Work out the finished part from the listing and answer in its coordinate system (mm). Coordinates: 2 decimals unless noted, no trailing zeros. Order: outer loops, then holes, each group sorted by start corner. A loop starts at its lowest first (then second) coordinate and runs counter-clockwise, first axis right, second up.
```python
from build123d import *

# Parameters (mm, degrees)
SKETCH_1_R      = 1.6
SKETCH_1_R_2    = 5.5
EXTRUDE_2_DEPTH = 2
FILLET_6_R      = 8
FILLET_7_R      = 8
FILLET_8_R      = 8
FILLET_9_R      = 8


with BuildPart() as part:
    # 草图1 → 凸台-拉伸2 (new body)
    # profile 1 of 2: a face of its own
    with BuildSketch(Plane.XY):
        with BuildLine():
            Line((-16.6, 15), (-19.5, 15))
            Line((-19.5, 15), (-19.5, -19.5))
            Line((-19.5, -19.5), (19.5, -19.5))
            Line((19.5, -19.5), (19.5, 19.5))
            Line((19.5, 19.5), (-15, 19.5))
            Line((-15, 19.5), (-15, 16.6))
            ThreePointArc((-15, 16.6), (-13.86862915, 16.13137085), (-13.4, 15))
            ThreePointArc((-13.4, 15), (-15, 13.4), (-16.6, 15))
        make_face()
        with Locations((-15, -15)):
            Circle(SKETCH_1_R, mode=Mode.SUBTRACT)
        with Locations((15, -15)):
            Circle(SKETCH_1_R, mode=Mode.SUBTRACT)
        Circle(SKETCH_1_R_2, mode=Mode.SUBTRACT)
        with Locations((15, 15)):
            Circle(SKETCH_1_R, mode=Mode.SUBTRACT)
    # profile 2 of 2: a face of its own
    with BuildSketch(Plane.XY):
        with BuildLine():
            Line((-19.5, 19.5), (-19.5, 15))
            Line((-19.5, 15), (-16.6, 15))
            ThreePointArc((-16.6, 15), (-16.13137085, 16.13137085), (-15, 16.6))
            Line((-15, 16.6), (-15, 19.5))
            Line((-15, 19.5), (-19.5, 19.5))
        make_face()
    extrude(amount=EXTRUDE_2_DEPTH)

    # 圆角6
    fillet_6_edges = [part.edges().sort_by_distance(p)[0] for p in [
        (-19.5, 19.5, 1),
    ]]
    fillet(fillet_6_edges, radius=FILLET_6_R)

    # 圆角7
    fillet_7_edges = [part.edges().sort_by_distance(p)[0] for p in [
        (19.5, 19.5, 1),
    ]]
    fillet(fillet_7_edges, radius=FILLET_7_R)

    # 圆角8
    fillet_8_edges = [part.edges().sort_by_distance(p)[0] for p in [
        (-19.5, -19.5, 1),
    ]]
    fillet(fillet_8_edges, radius=FILLET_8_R)

    # 圆角9
    fillet_9_edges = [part.edges().sort_by_distance(p)[0] for p in [
        (19.5, -19.5, 1),
    ]]
    fillet(fillet_9_edges, radius=FILLET_9_R)


solid = part.part
```
1. Consider probe 1 along Y at (x, z) = (0, 0.95); probe 2 along Y at (x, z) = (15, 1.45); probe 3 along X at (y, z) = (16, 1.35). Determine where each line is inside the solid, lowest interval first.
2. The mould has two halves that part along X. Classify faces 1 (the cylindrical face through (17.094, 17.219, 1.014)), 2 (the cylindrical face through (13.4, 15.07, 0.99)), 3 (the cylindrical face through (-17.219, 17.094, 1.014)): released by +X, released by -X, zero draft, split by the parting line, or undercut.
3. The part is cut by section B-B (z = 0.5). Determine the outline of the cut face in (x, y).
4. The part is cut by section D-D (x = 14.5). Determine the outline of the cut face in (y, z), plus the area to 3 significant figures.
5. The part is cut by section A-A (x = 0). Determine the outline of the cut face in (y, z), plus the area to 3 significant figures.
Worked out:
1. probe 1: y = -19.5 to -5.5, 5.5 to 19.5
1. probe 2: y = -18.69 to -16.6, -13.4 to 13.4, 16.6 to 18.69
1. probe 3: x = -18.11 to -16.25, -13.75 to 13.75, 16.25 to 18.11
2. face 1: released by +X
2. face 2: undercut
2. face 3: released by -X
3. outline: (-19.5, -11.5) arc R8 ccw to (-11.5, -19.5) - (11.5, -19.5) arc R8 ccw to (19.5, -11.5) - (19.5, 11.5) arc R8 ccw to (11.5, 19.5) - (-11.5, 19.5) arc R8 ccw to (-19.5, 11.5) - close; hole circle Ø3.2 at (-15, -15); hole circle Ø3.2 at (-15, 15); hole circle Ø11 at (0, 0); hole circle Ø3.2 at (15, -15); hole circle Ø3.2 at (15, 15)
4. outline: (-18.92, 0) - (-16.52, 0) - (-16.52, 2) - (-18.92, 2) - close; (-13.48, 0) - (13.48, 0) - (13.48, 2) - (-13.48, 2) - close; (16.52, 0) - (18.92, 0) - (18.92, 2) - (16.52, 2) - close
4. area: 63.5 mm2
5. outline: (-19.5, 0) - (-5.5, 0) - (-5.5, 2) - (-19.5, 2) - close; (5.5, 0) - (19.5, 0) - (19.5, 2) - (5.5, 2) - close
5. area: 56.0 mm2
